Autodesk Inventor part; units mm, degrees
ref_plane "Work Plane1" through (21, 8.7, 8.75) normal (1, 0, 0) x (0, 0, -1)
ref_plane "YZ Plane" through (0, 0, 0) normal (1, 0, 0) x (0, 1, 0)
ref_plane "XZ Plane" through (0, 0, 0) normal (0, 1, 0) x (-1, 0, 0)
sketch "Sketch2" plane through (0, 0, 0) normal (0, 0, 1) x (1, 0, 0)
  line L0 (0, 0) -> (42, 0)
  line L1 (42, 0) -> (42, 32)
  line L2 (42, 32) -> (0, 32)
  line L3 (0, 32) -> (0, 0)
  dimension "d0" = 42
  dimension "d1" = 32
extrude "Servo_Housing" add sketch "Sketch2" along normal blind 15
sketch "Sketch4" plane through (0, 0, 15) normal (0, 0, 1) x (1, 0, 0)
  line L0 (42, 32) -> (0, 32)
  line L1 (0, 32) -> (0, 0)
  line L2 (4.5, 24.7) -> (9.5, 24.7)
  line L3 (9.5, 24.7) -> (9.5, 8.7)
  line L4 (9.5, 8.7) -> (32.5, 8.7)
  line L5 (32.5, 8.7) -> (32.5, 24.7)
  line L6 (32.5, 24.7) -> (37.5, 24.7)
  line L7 (42, 0) -> (42, 32)
  line L8 (0, 0) -> (42, 0)
  line L9 (4.5, 24.7) -> (4.5, 27)
  line L10 (4.5, 27) -> (9.5, 27)
  line L11 (9.5, 27) -> (9.5, 32)
  line L12 (37.5, 27) -> (37.5, 24.7)
  line L13 (37.5, 27) -> (32.5, 27)
  line L14 (32.5, 27) -> (32.5, 32)
  line L15 (9.5, 32) -> (32.5, 32)
  line L16 (21, 36.5125) -> (21, -47.625) construction
  point P0 (4.9935, 32)
  point P1 (37, 32)
  dimension "d6" = 5
  dimension "d7" = 16
  dimension "d8" = 23
  dimension "d11" = 8.7
  dimension "d14" = 2.3
  dimension "d15" = 2.3
  dimension "d22" = 42
  dimension "d23" = 21
  dimension "d24" = 23
  dimension "d25" = 11.5
  dimension "d26" = 5
  dimension "d27" = 5
  dimension "d28" = 5
extrude "Servo_Opening" cut sketch "Sketch4" against normal blind 6.25 contours L14 L13 L12 L6 L5 L4 L3 L2 L9 L10 L11 L0
sketch "Sketch5" plane through (0, 0, 15) normal (0, 0, 1) x (1, 0, 0)
  line L0 (42, 0) -> (42, 32)
  line L1 (42, 14.7) -> (42, 13.2)
  line L2 (-29.647, 13.95) -> (54.8226, 13.95) construction
  line L3 (0, 0) -> (42, 0)
  line L4 (32.5, 8.7) -> (9.5, 8.7)
  line L5 (42, 13.2) -> (32.5, 13.2)
  line L6 (32.5, 13.2) -> (32.5, 14.7)
  line L7 (32.5, 24.7) -> (32.5, 8.7)
  line L8 (42, 14.7) -> (32.5, 14.7)
  dimension "d171" = 1.5
  dimension "d211" = 4.5
extrude "Cable_Opening" cut sketch "Sketch5" against normal blind 2.5
sketch "Sketch6" plane through (0, 0, 15) normal (0, 0, 1) x (1, 0, 0)
  circle A0 centre (3.5, 28) radius 1.1
  circle A1 centre (38.5, 28) radius 1.1
  circle A2 centre (38.5, 4) radius 1.1
  circle A3 centre (3.5, 4) radius 1.1
  line L0 (21, 34.35) -> (21, -13.275) construction
  line L1 (-20.6375, 16) -> (66.675, 16) construction
  line L2 (42, 14.7) -> (42, 32)
  line L3 (0, 32) -> (0, 0)
  line L4 (9.5, 32) -> (0, 32)
  line L5 (0, 0) -> (42, 0)
  point P0 (42, 12.35)
  point P1 (0, 12.35)
  dimension "d29" = 2.2
  dimension "d30" = 2.2
  dimension "d31" = 2.2
  dimension "d32" = 2.2
  dimension "d33" = 42
  dimension "d34" = 21
  dimension "d35" = 32
  dimension "d36" = 16
  dimension "d37" = 35
  dimension "d38" = 17.5
  dimension "d39" = 24
  dimension "d40" = 12
extrude "Cover_Mounting_Holes" cut sketch "Sketch6" against normal up to surface (15 mm away)
sketch "Sketch10" plane through (0, 0, 15) normal (0, 0, 1) x (1, 0, 0)
  line L0 (32.5, 8.7) -> (9.5, 8.7)
  line L1 (9.5, 8.7) -> (32.5, 8.7)
  line L2 (32.5, 8.7) -> (32.5, 0)
  line L3 (32.5, 0) -> (9.5, 0)
  line L4 (9.5, 0) -> (9.5, 8.7)
  line L5 (9.5, 8.7) -> (9.5, 24.7)
  line L6 (32.5, 24.7) -> (32.5, 14.7)
  point P0 (0, 0)
  point P1 (9.5, 12.35)
  point P2 (32.5, 12.35)
extrude "Pin" add sketch "Sketch10" along normal blind 5.8
sketch "Sketch11" plane through (9.5, 8.7, 8.75) normal (0, 1, 0) x (1, 0, 0)
  circle A0 centre (17.2, -6.25) radius 1.6
  line L0 (-9.5, -6.05) -> (-9.5, -3.55)
  line L1 (32.5, 8.75) -> (32.5, -6.25)
  point P0 (-9.5, 8.75)
  point P1 (0, -6.25)
  dimension "d65" = 3.2
  dimension "d69" = 15.3
extrude "Shaft_Opening" cut sketch "Sketch11" against normal up to surface (8.7 mm away)
sketch "Sketch12" plane through (9.5, 8.7, 8.75) normal (0, 1, 0) x (1, 0, 0)
  circle A0 centre (17.2, -6.25) radius 4
  circle A1 centre (17.2, -6.25) radius 1.6
  point P0 (-9.5, 8.75)
  dimension "d73" = 8
extrude "Nut_Slot" cut sketch "Sketch12" against normal blind 5.7
sketch "Sketch15" plane through (0, 0, 15) normal (0, 0, 1) x (1, 0, 0)
  line L0 (9.5, 32) -> (0, 32)
  line L1 (0, 0) -> (9.5, 0)
  line L2 (39, 24.5) -> (42, 24.5)
  line L3 (42, 32) -> (32.5, 32)
  line L4 (42, 5.5) -> (39, 5.5)
  line L5 (32.5, 0) -> (42, 0)
  line L6 (42, 32) -> (0, 32)
  line L7 (0, 32) -> (0, 42)
  line L8 (0, 42) -> (-21.8, 42)
  line L9 (0, 32) -> (6, 32)
  line L10 (6, 32) -> (6, 49.5)
  line L11 (6, 49.5) -> (-26.8, 49.5)
  line L12 (0, 0) -> (0, -10)
  line L13 (0, -10) -> (-21.8, -10)
  line L14 (-21.8, -10) -> (-21.8, 42)
  line L15 (0, 0) -> (6, 0)
  line L16 (6, 0) -> (6, -17.5)
  line L17 (6, -17.5) -> (-26.8, -17.5)
  line L18 (-26.8, -17.5) -> (-26.8, 49.5)
  line L19 (0, 32) -> (0, 0)
  point P0 (0, 5.5)
  dimension "d111" = 10
  dimension "d113" = 6
  dimension "d114" = 17.5
  dimension "d116" = 10
  dimension "d117" = 21.8
  dimension "d118" = 6
  dimension "d119" = 17.5
  dimension "d120" = 32.8
  dimension "d161" = 7.5
  dimension "d175" = 32.8
  dimension "d191" = 5
extrude "Connection_Adapter" add sketch "Sketch15" along normal mid plane 30 contours L0 L7 L8 L14 L13 L12 L1 L16 L17 L18 L11 L10
sketch "Sketch17" plane through (-21.8, -10, 30) normal (1, 0, 0) x (0, 0, -1)
  circle A0 centre (15, 26) radius 11 construction
  line L0 (30, 52) -> (0, 52)
  line L1 (30, 0) -> (0, 0)
  line L2 (0, 0) -> (0, 52)
  line L3 (30, 52) -> (30, 0)
  line L4 (15, 12.642) -> (15, 38.042) construction
  line L5 (1.1452, 26) -> (27.1241, 26) construction
  line L6 (4.9901, 15.9901) -> (35.9566, 46.9566) construction
  line L7 (5.2574, 35.7426) -> (22.7782, 18.2218) construction
  circle A1 centre (7.2218, 18.2218) radius 1.5
  circle A2 centre (4, 26) radius 1.5
  circle A3 centre (7.2218, 33.7782) radius 1.5
  circle A4 centre (15, 37) radius 1.5
  circle A5 centre (15, 15) radius 1.5
  circle A6 centre (22.7782, 18.2218) radius 1.5
  circle A7 centre (26, 26) radius 1.5
  circle A8 centre (22.7782, 33.7782) radius 1.5
  point P0 (30, 10)
  dimension "d121" = 22
  dimension "d122" = 52
  dimension "d123" = 26
  dimension "d124" = 30
  dimension "d125" = 15
  dimension "d126" = 3
  dimension "d127" = 3
  dimension "d128" = 3
  dimension "d129" = 3
  dimension "d130" = 3
  dimension "d131" = 3
  dimension "d132" = 3
  dimension "d133" = 3
  dimension "d134" = 45
  dimension "d135" = 45
extrude "Docking_Holes_Front" cut sketch "Sketch17" against normal up to surface (5 mm away) contours A1 | A2 | A3 | A4 | A5 | A6 | A7 | A8
sketch "Sketch19" plane through (-21.8, -10, 30) normal (1, 0, 0) x (0, 0, -1)
  circle A0 centre (15, 26) radius 5
  line L0 (30, 0) -> (0, 0)
  line L1 (30, 52) -> (0, 52)
  line L2 (30, 52) -> (30, 0)
  line L3 (0, 0) -> (0, 52)
  point P0 (30, 10)
  dimension "d140" = 10
  dimension "d141" = 52
  dimension "d142" = 26
  dimension "d143" = 30
  dimension "d144" = 15
extrude "Cable_Opening_Front" cut sketch "Sketch19" against normal up to surface (5 mm away) contours A0
sketch "Sketch22" plane through (0, 0, 0) normal (0, 0, -1) x (-1, 0, 0)
  circle A0 centre (-38.5, 28) radius 1.1
  line L0 (-39.6, 28) -> (-2.4, 28) construction
  circle A1 centre (-3.5, 28) radius 1.1
  line L1 (-3.5, 36.8375) -> (-3.5, -9.2) construction
  circle A2 centre (-38.5, 4) radius 1.1
  line L2 (-39.6, 4) -> (-2.2922, 4) construction
  line L3 (-42, 0) -> (-42, 32)
  line L4 (0, -10) -> (0, 42)
  line L5 (-6, 0) -> (-42, 0)
  line L6 (-42, 32) -> (-6, 32)
  circle A3 centre (-3.5, 28) radius 1.6
  circle A4 centre (-3.5, 28) radius 1.1
  circle A5 centre (-3.5, 4) radius 1.6
  circle A6 centre (-38.5, 28) radius 1.6
  circle A7 centre (-38.5, 4) radius 1.6
  circle A8 centre (-38.5, 4) radius 1.1
  circle A9 centre (-3.5, 4) radius 1.1
  circle A10 centre (-38.5, 28) radius 1.1
  point P0 (0, 0)
  point P1 (0, -1)
  point P2 (0, 33)
  dimension "d166" = 3.2
  dimension "d167" = 3.2
  dimension "d168" = 3.2
  dimension "d169" = 3.2
  dimension "d176" = 2.4
  dimension "d177" = 1.9
extrude "Insert_Opening" cut sketch "Sketch22" against normal blind 5
fillet "Fillet4" radius 8 2 edges at (0, 42, 15) (0, -10, 15)
chamfer "Chamfer1" distance 12 angle 18 1 edges at (6, -8.75, 30) measured on face at (6, -11.6667, 15)
chamfer "Chamfer2" distance 12 angle 18 1 edges at (6, -8.75, 0) measured on face at (6, -11.6667, 11)
chamfer "Chamfer3" distance 12 angle 18 1 edges at (6, 40.75, 30) measured on face at (6, 43.6667, 15)
chamfer "Chamfer4" distance 12 angle 18 1 edges at (6, 40.75, 0) measured on face at (6, 43.6667, 11)
fillet "Fillet5" radius 5 2 edges at (-21.8, -10, 15) (-21.8, 42, 15)
sketch "Sketch24" plane through (0, 0, 8.75) normal (0, 0, 1) x (1, 0, 0)
  circle A0 centre (14.75, 26.6) radius 1.75
  line L0 (9.5, 32) -> (32.5, 32)
  line L1 (9.5, 27) -> (9.5, 32)
  line L2 (32.5, 32) -> (32.5, 27)
  point P0 (0, 0)
  dimension "d192" = 3.5
  dimension "d193" = 5.4
  dimension "d194" = 5.25
  dimension "d200" = 23
extrude "Heat_dissipation_Hole" cut sketch "Sketch24" against normal up to surface (8.75 mm away)
pattern_linear "Rectangular Pattern1" count 3 spacing 6.25 along (1, 0, 0) count 3 spacing 6.25 along (0, -1, 0) of "Heat_dissipation_Hole"
sketch "Sketch25" plane through (-26.8, -17.5, 0) normal (0, -1, 0) x (1, 0, 0)
  line L0 (10, 22.5) -> (18.8, 22.5)
  line L1 (18.8, 22.5) -> (18.8, 7.5)
  line L2 (18.8, 7.5) -> (10, 7.5)
  line L3 (10, 7.5) -> (10, 22.5)
  line L4 (0, 30) -> (28.901, 30)
  line L5 (0, 0) -> (0, 30)
  point P0 (26.8, 0)
  dimension "d204" = 8.8
  dimension "d205" = 15
  dimension "d206" = 7.5
  dimension "d207" = 10
extrude "Extrusion22" [suppressed]
fillet "Fillet6" [suppressed]
ref_plane "Work Plane1" through (21, 8.7, 8.75) normal (1, 0, 0) x (0, 0, -1)
equation "\"d15\" = d14"
equation "\"d23\" = 0.5 * d22"
equation "\"d25\" = 0.5 * d24"
equation "\"d27\" = d26"
equation "\"d28\" = d6"
equation "\"d34\" = 0.5 * d33"
equation "\"d36\" = 0.5 * d35"
equation "\"d38\" = 0.5 * d37"
equation "\"d40\" = 0.5 * d39"
equation "\"d65\" = d70"
equation "\"d142\" = 0.5 * d141"
equation "\"d144\" = 0.5 * d143"
equation "\"d166\" = d168"
equation "\"d167\" = d168"
equation "\"d169\" = d168"
properties part number "Module_Body"
CAD build for the part. Positions are in the model's coordinates, mm. A direction names the side the tool comes from. Coordinates: 2 decimals unless noted, no trailing zeros. Order: outer loops, then holes, each group sorted by start corner. A loop starts at its lowest first (then second) coordinate and runs counter-clockwise, first axis right, second up. Notation, with made-up numbers: M 81,-13.75 L 108,-13.75 A20 ccw 108,21.25 Z; hole C 61.25,-36.75 d4. An arc over 180 degrees is marked long. Answer as CSV lines item,"result".
1) Drill centre lines: L1, parallel to Y at x = 38.5, z = 3.2; L2, parallel to Y at x = 38.5, z = 10.5; L3, parallel to Y at x = 27.25, z = 6.75. Where is each one in solid material? Low to high. Write a range as from..to.
Verdict:
L1,"0..2.4, 5.6..26.4, 29.6..32"
L2,"0..2.9, 5.1..26.9, 29.1..32"
L3,"0..12.35, 15.85..18.6, 22.1..24.85, 28.35..32"
2) Flat gauge pins, fed straight in: P1, Ø4, axis at y = -4, z = 13.5, coming from the +X side; P2, Ø1.5, axis at x = 32.5, y = 28, coming from the +Z side; P3, Ø5.5, axis at x = 35.5, z = 12, coming from the +Y side. Where does each tip first touch, or does it go through?
Verdict:
P1,"x = 6"
P2,"z = 15"
P3,"y = 32"
3) 3-axis set-ups, long thin cutter, end or side, ignore diameter. For faces 1 (the flat face through (4.023, 40.872, 5.916)), 2 (the flat face through (0, 16, 8)), 3 (the cylindrical face through (37.76, 2.58, 2.46)): which of +Z, -Z, +X, -X, +Y, -Y reach the whole face in a straight line?
Verdict:
face 1,"-Z, +X, +Y"
face 2,"+Z, -Z"
face 3,"-Z"
4) Cut at B-B (y = -3). List the corners of the cut face in (x, z).
Verdict:
outline,"M -26.8,0 L -21.8,0 L -21.8,30 L -26.8,30 Z; M -0.06,0 L 2.1,0 L 6,12 L 6,18 L 2.1,30 L -0.06,30 Z"
5) Mould opens along Y. For faces 4 (the flat face through (-12, -10, 15)), 5 (the flat face through (37, 7, 15)), 6 (the flat face through (-10, 49.5, 15)) say: released by +Y, released by -Y, zero draft, split by the parting line, or undercut.
Verdict:
face 4,"undercut"
face 5,"zero draft"
face 6,"released by +Y"
6) Cut at D-D (z = 4). Give the number of separate pieces and of enclosed holes in the cut face, then the cut area to 3 significant figures.
Verdict:
separate pieces,"1"
enclosed holes,"13"
area,"2,030 mm2"
7) Cut at A-A (x = 21). List the corners of the cut face in (y, z), then the cut area to 3 significant figures.
Verdict:
outline,"M 0,0 L 12.35,0 L 12.35,8.75 L 8.7,8.75 L 8.7,20.8 L 0,20.8 Z; M 15.85,0 L 18.6,0 L 18.6,8.75 L 15.85,8.75 Z; M 22.1,0 L 24.85,0 L 24.85,8.75 L 22.1,8.75 Z; M 28.35,0 L 32,0 L 32,8.75 L 28.35,8.75 Z"
area,"293 mm2"
8) Cut at C-C (x = -11.5). List the corners of the cut face in (y, z), then the cut area to 3 significant figures.
Verdict:
outline,"M -17.5,0 L -10,0 L -10,30 L -17.5,30 Z; M 42,0 L 49.5,0 L 49.5,30 L 42,30 Z"
area,"450 mm2"
